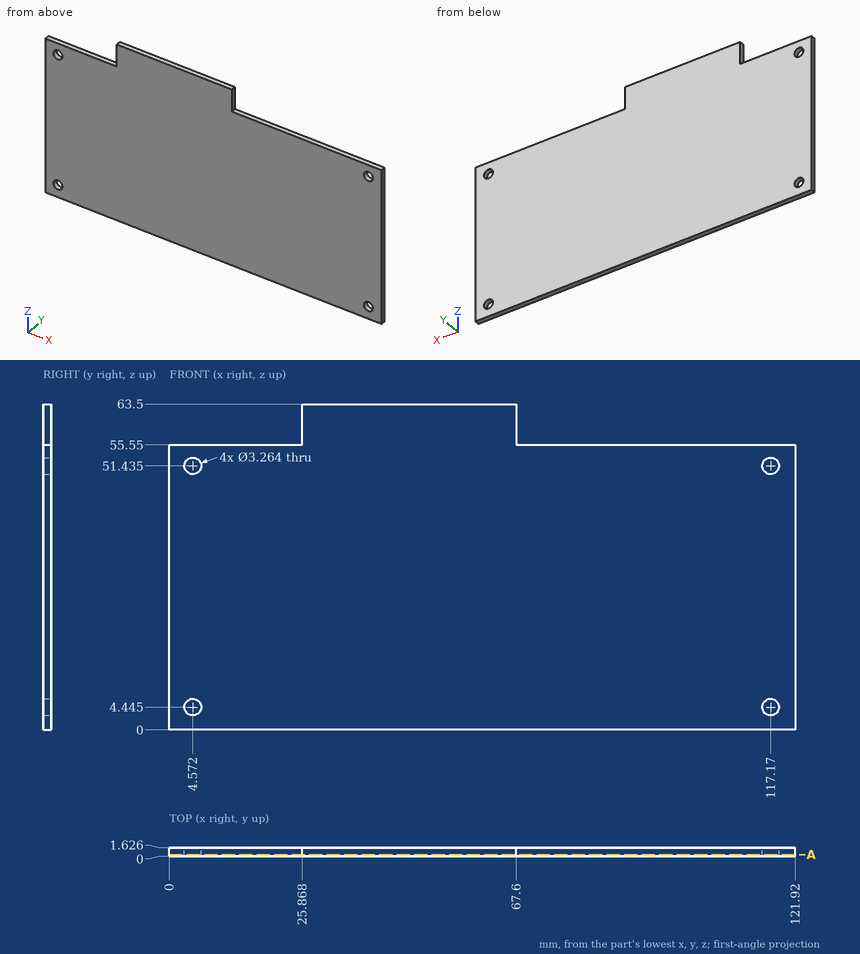
Can you work these out from the drawing? Everything is in mm from the part's minimum corner. Give positions to 0.01 mm unless a question says otherwise; leave off trailing zeros. Return JSON: item names as keys, results as strings.
1. Imagine slicing it at A-A on y = 0.3. Give the number of separate pieces and of enclosed holes in the cut face, then the cut area to 3 significant figures.
Answer list:
{"separate pieces": "1", "enclosed holes": "4", "area": "7,070 mm2"}
2. For pin 1 Ø8 at (x, z) = (93.5, 23) entering from -Y; pin 2 Ø2 at (x, z) = (117.17, 51.44) entering from -Y; pin 3 Ø0.8 at (x, y) = (17, 1) entering from +Z, each with a flat end and sliding along its axis, tell me the tip position at first contact or that it passes through.
Answer list:
{"pin 1": "stops at y = 0", "pin 2": "passes through", "pin 3": "stops at z = 55.55"}
3. I need wall thicknesses on line 1 (X direction, y = 1.35, z = 3.5); line 2 (Z direction, x = 116, y = 1.55); line 3 (Z direction, x = 105, y = 1.3). Which ranges of each line are inside material? Lowest first, please. Write a range as from..to.
Answer list:
{"line 1": "x = 0..3.24, 5.9..115.84, 118.5..121.92", "line 2": "z = 0..3.31, 5.58..50.3, 52.57..55.55", "line 3": "z = 0..55.55"}
